from build123d import *

# Parameters (mm, degrees)
SKETCH_W        = 180
SKETCH_H        = 180
SKETCH_W_2      = 170.5
SKETCH_H_2      = 170.5
PAD_DEPTH       = 30
CHAMFER_SIZE    = 15
SKETCH001_W     = 120
SKETCH001_H     = 120
PAD001_DEPTH    = 5
SKETCH002_W     = 143
SKETCH002_H     = 30
POCKET_DEPTH    = 10
SKETCH003_R     = 2.5
POCKET001_DEPTH = 35.001
CHAMFER001_SIZE = 4
CHAMFER002_SIZE = 4


with BuildPart() as part:
    # Sketch → Pad (new body)
    with BuildSketch(Plane.XY):
        Rectangle(SKETCH_W, SKETCH_H)
        Rectangle(SKETCH_W_2, SKETCH_H_2, mode=Mode.SUBTRACT)
    extrude(amount=PAD_DEPTH)

    # Chamfer
    chamfer_edges = [part.edges().sort_by_distance(p)[0] for p in [
        (-90, -90, 15),
        (-85.25, -85.25, 15),
        (-85.25, 85.25, 15),
        (-90, 90, 15),
        (85.25, 85.25, 15),
        (90, 90, 15),
        (85.25, -85.25, 15),
        (90, -90, 15),
    ]]
    chamfer(chamfer_edges, length=CHAMFER_SIZE)

    # Sketch001 (on Face5 of Chamfer) → Pad001 (join)
    with BuildSketch(Plane.XY.offset(30)):
        Polygon((-90, -75), (-90, 75), (-75, 90), (-71.5, 90), (-71.5, 98), (71.5, 98), (71.5, 90), (75, 90), (90, 75), (90, -75), (75, -90), (-75, -90), align=None)
        Rectangle(SKETCH001_W, SKETCH001_H, mode=Mode.SUBTRACT)
    extrude(amount=PAD001_DEPTH)

    # Sketch002 (on Face24 of Pad001) → Pocket (cut)
    with BuildSketch(Plane(origin=(0, 90, 0), x_dir=(-1, 0, 0), z_dir=(0, 1, 0))):
        with Locations((0, 15)):
            Rectangle(SKETCH002_W, SKETCH002_H)
    extrude(amount=-POCKET_DEPTH, mode=Mode.SUBTRACT)

    # Sketch003 (on Face20 of Pocket) → Pocket001 (cut, through all)
    with BuildSketch(Plane.XY.offset(35)):
        with Locations((-50, 89)):
            Circle(SKETCH003_R)
        with Locations((50, 89)):
            Circle(SKETCH003_R)
    extrude(amount=-POCKET001_DEPTH, mode=Mode.SUBTRACT)

    # Chamfer001
    chamfer001_edges = [part.edges().sort_by_distance(p)[0] for p in [
        (90, 0, 35),
        (82.5, -82.5, 35),
        (0, -90, 35),
        (-82.5, -82.5, 35),
        (-90, 0, 35),
    ]]
    chamfer(chamfer001_edges, length=CHAMFER001_SIZE)

    # Chamfer002
    chamfer002_edges = [part.edges().sort_by_distance(p)[0] for p in [
        (82.5, 82.5, 0),
        (90, 0, 0),
        (82.5, -82.5, 0),
        (0, -90, 0),
        (-82.5, -82.5, 0),
        (-90, 0, 0),
        (-82.5, 82.5, 0),
    ]]
    chamfer(chamfer002_edges, length=CHAMFER002_SIZE)


solid = part.part
Here's how the part is built. I have some questions about the finished solid (model axes, mm). A direction names the side the tool comes from. Round coordinates to 2 decimals unless told otherwise and drop trailing zeros. Write each loop counter-clockwise with the first axis right and the second up, starting at its lowest first coordinate (ties: lowest second). Pieces come first, ordered by that corner, then holes.
1. For faces 4 (the flat face through (-78.5, 77, 14.8)), 5 (the flat face through (71.5, 87, 15)), 6 (the flat face through (-60, -1, 32)), which set-ups out of +Z, -Z, +X, -X, +Y, -Y let a thin tool reach every point of the face, with its end or its side?
2. Suppose I cut it at A-A (x = 3.5). List the corners of the cut face in (y, z) for me.
3. If we mould it in two halves opening along Y, with no side actions, what happens to faces 1 (the flat face through (88, 3, 33)), 2 (the flat face through (85.25, -1, 15)), 3 (the flat face through (-81, -81.21, 32.97))? For each: released by +Y, released by -Y, zero draft, split by the parting line, or undercut.
4. I need wall thicknesses on L1, parallel to Y at x = -50, z = 31; L2, parallel to X at y = -46, z = 14; L3, parallel to Y at x = -50, z = 32.1. Which ranges of each line are inside material? Lowest first, please.
5. Suppose I cut it at B-B (y = 18). List the corners of the cut face in (x, z) for me, and give its area (3 significant figures).
6. Will these pins go through, and if not, where does the flat tip stop? pin 1 Ø1 at (x, z) = (-74, 19) entering from +Y; pin 2 Ø5 at (y, z) = (86.5, 13.5) entering from +X; pin 3 Ø5.5 at (y, z) = (96, 32.5) entering from -X.
7. Suppose I cut it at D-D (x = -50). List the corners of the cut face in (y, z) for me.
8. Suppose I cut it at C-C (z = 11.5). List the corners of the cut face in (x, y) for me, and give its area (3 significant figures).
Answer sheet:
1. face 4: -Z
1. face 5: -Z, +Y
1. face 6: +Z, -Z
2. outline: (-90, 4) - (-86, 0) - (-85.25, 0) - (-85.25, 30) - (-60, 30) - (-60, 35) - (-86, 35) - (-90, 31) - close; (60, 30) - (98, 30) - (98, 35) - (60, 35) - close
3. face 1: zero draft
3. face 2: undercut
3. face 3: released by -Y
4. L1: y = -90 to -60, 60 to 86.5, 91.5 to 98
4. L2: x = -90 to -85.25, 85.25 to 90
4. L3: y = -88.9 to -60, 60 to 86.5, 91.5 to 98
5. outline: (-90, 4) - (-86, 0) - (-85.25, 0) - (-85.25, 30) - (-60, 30) - (-60, 35) - (-86, 35) - (-90, 31) - close; (60, 30) - (85.25, 30) - (85.25, 0) - (86, 0) - (90, 4) - (90, 31) - (86, 35) - (60, 35) - close
5. area: 553 mm2
6. pin 1: stops at y = 90
6. pin 2: stops at x = 81
6. pin 3: stops at x = -71.5
7. outline: (-90, 4) - (-86, 0) - (-85.25, 0) - (-85.25, 30) - (-60, 30) - (-60, 35) - (-86, 35) - (-90, 31) - close; (60, 30) - (86.5, 30) - (86.5, 35) - (60, 35) - close; (91.5, 30) - (98, 30) - (98, 35) - (91.5, 35) - close
8. outline: (-90, -75) - (-75, -90) - (75, -90) - (90, -75) - (90, 75) - (75, 90) - (71.5, 90) - (71.5, 84) - (85.25, 70.25) - (85.25, -70.25) - (70.25, -85.25) - (-70.25, -85.25) - (-85.25, -70.25) - (-85.25, 70.25) - (-71.5, 84) - (-71.5, 90) - (-75, 90) - (-90, 75) - close
8. area: 2,650 mm2
